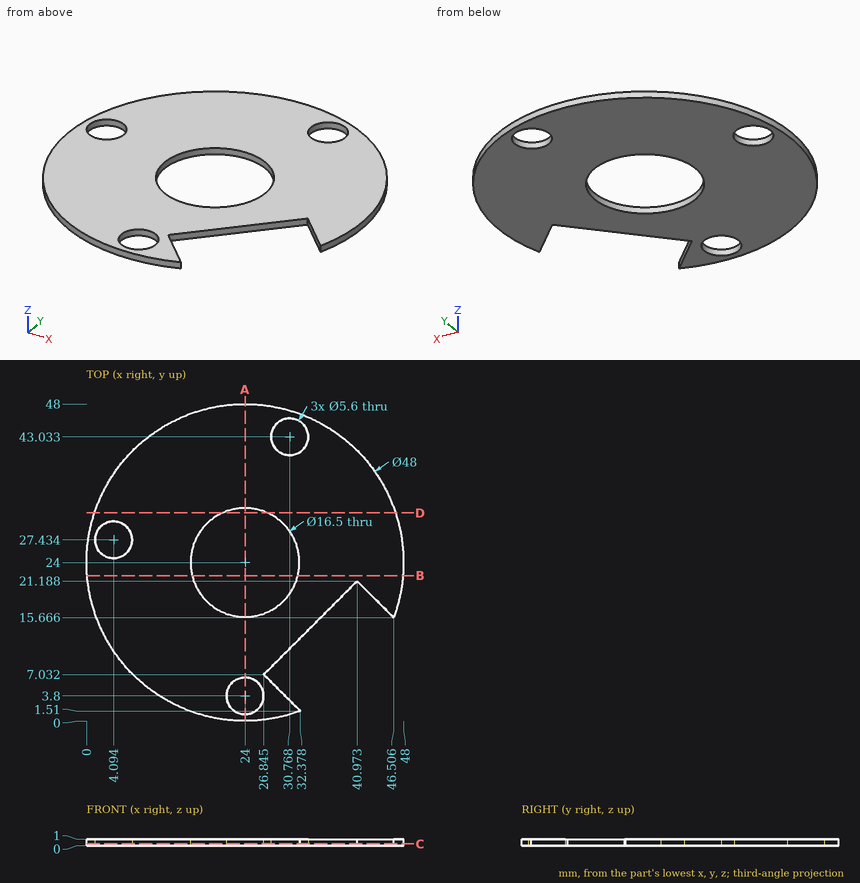
Answer from the drawing. Dimensions are ordinates in mm from the lowest x, y and z of the part. Coordinates: 2 decimals unless noted, no trailing zeros. Order: outer loops, then holes, each group sorted by start corner. A loop starts at its lowest first (then second) coordinate and runs counter-clockwise, first axis right, second up. Notation, with made-up numbers: (78, 81.5) - (95, 81.5) arc R5 cw to (95, 87.5) - close; hole circle Ø8 at (60.5, 47.25). An arc over 180 degrees is marked (long way). Put each result on its own line as item: value. Start each with the question number.
1) Find section D-D (y = 31.5). Give the vertices of the cut face in (x, z).
2) Find section C-C (z = 0.25). State how many separate pieces and enclosed holes the cut face has, plus the area to 3 significant figures.
3) Find section A-A (x = 24). Give the vertices of the cut face in (y, z).
4) Find the intervals of material crossed by line 1 (Y direction, x = 24, z = 0.25); line 2 (X direction, y = 24, z = 0.4); line 3 (X direction, y = 26, z = 0.75) (1 decimal), in increasing order. Write a range as from..to.
5) Find section B-B (y = 22). Give the vertices of the cut face in (x, z).
Results list:
1. outline: (1.2, 0) - (20.56, 0) - (20.56, 1) - (1.2, 1) - close; (27.44, 0) - (46.8, 0) - (46.8, 1) - (27.44, 1) - close
2. separate pieces: 1
2. enclosed holes: 4
2. area: 1,340 mm^2
3. outline: (0, 0) - (1, 0) - (1, 1) - (0, 1) - close; (6.6, 0) - (15.75, 0) - (15.75, 1) - (6.6, 1) - close; (32.25, 0) - (48, 0) - (48, 1) - (32.25, 1) - close
4. line 1: y = 0..1, 6.6..15.75, 32.25..48
4. line 2: x = 0..15.75, 32.25..48
4. line 3: x = 0.1..1.7, 6.5..16, 32..47.9
5. outline: (0.08, 0) - (16, 0) - (16, 1) - (0.08, 1) - close; (32, 0) - (47.92, 0) - (47.92, 1) - (32, 1) - close
